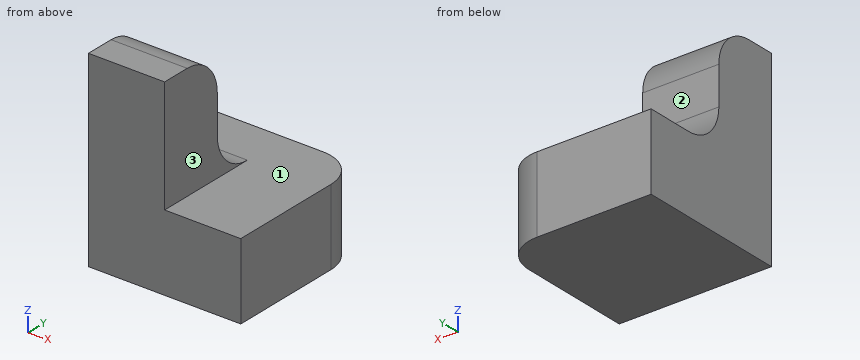
```python
from build123d import *

# Parameters (mm, degrees)
SKETCH1_W           = 20
SKETCH1_H           = 17.5
BOSS_EXTRUDE1_DEPTH = 30
SKETCH2_W           = 40
SKETCH2_H           = 40
BOSS_EXTRUDE2_DEPTH = 20
FILLET1_R           = 10


with BuildPart() as part:
    # Sketch1 → Boss-Extrude1 (new body)
    with BuildSketch(Plane.XY):
        with Locations((-20, -8.75)):
            Rectangle(SKETCH1_W, SKETCH1_H)
    extrude(amount=BOSS_EXTRUDE1_DEPTH)

    # Sketch2 → Boss-Extrude2 (add)
    with BuildSketch(Plane.XY):
        with Locations((-10, 2.5)):
            Rectangle(SKETCH2_W, SKETCH2_H)
    extrude(amount=-BOSS_EXTRUDE2_DEPTH)

    # Fillet1
    fillet1_edges = [part.edges().sort_by_distance(p)[0] for p in [
        (10, 22.5, -10),
        (-20, 0, 30),
        (-20, 0, 0),
    ]]
    fillet(fillet1_edges, radius=FILLET1_R)


solid = part.part
```
Design review of the part built by this model. Coordinates are the model's own, in mm. Face numbers are marked on the shaded views. A direction names the side the tool comes from. Coordinates: 2 decimals unless noted, no trailing zeros. Order: outer loops, then holes, each group sorted by start corner. A loop starts at its lowest first (then second) coordinate and runs counter-clockwise, first axis right, second up.
1) Take a section at A-A, the plane x = -25.5. Give the boundary of the cut face in (y, z), and give its area (4 significant figures).
2) For the marked faces 1, 2 and 3, list the 3-axis set-ups (+Z, -Z, +X, -X, +Y, -Y) from which the entire face can be reached by the end or side of a thin tool; tool diameter is ignored.
3) Take a section at D-D, the plane x = -5. Give the boundary of the cut face in (y, z).
4) Take a section at C-C, the plane z = 14.5. Give the boundary of the cut face in (x, y).
5) Take a section at B-B, the plane y = -14.5. Give the boundary of the cut face in (x, z), and give its area (3 significant figures).
6) Wall thickness on line 1 along Z through (x, y) = (4, 1.5); line 2 along X through (y, z) = (-6.5, 8); line 3 along Z through (x, y) = (-13, -7): over which ranges is each line inside the solid? List them lowest first.
7) Clearance check with flat-ended pins moving along their axes: pin 1 (8 mm diameter, centred on y = -2, z = 17, fed in from +X); pin 2 (1.5 mm diameter, centred on x = -17, y = 5, fed in from +Z); pin 3 (6 mm diameter, centred on x = -9, z = 21, fed in from +Y). State where each tip first meets the part, or that it passes through.
Returned:
1. outline: (-17.5, -20) - (22.5, -20) - (22.5, 0) - (10, 0) arc R10 cw to (0, 10) - (0, 20) arc R10 ccw to (-10, 30) - (-17.5, 30) - close
1. area: 1,325 mm2
2. face 1: +Z, +X, +Y
2. face 2: +Z, +X, -X, +Y
2. face 3: +Z, +X, +Y, -Y
3. outline: (-17.5, -20) - (22.5, -20) - (22.5, 0) - (-17.5, 0) - close
4. outline: (-30, -17.5) - (-10, -17.5) - (-10, 0) - (-30, 0) - close
5. outline: (-30, -20) - (10, -20) - (10, 0) - (-10, 0) - (-10, 30) - (-30, 30) - close
5. area: 1,400 mm2
6. line 1: z = -20 to 0
6. line 2: x = -30 to -10
6. line 3: z = -20 to 29.54
7. pin 1: stops at x = -10
7. pin 2: stops at z = 1.82
7. pin 3: stops at y = 0
